```python
from build123d import *

# Parameters (mm, degrees)
SKETCH1_R           = 57
BOSS_EXTRUDE1_DEPTH = 38
SKETCH2_R           = 51
CUT_EXTRUDE1_DEPTH  = 39
SKETCH4_R           = 1.5
CUT_EXTRUDE3_DEPTH  = 15


with BuildPart() as part:
    # Sketch1 → Boss-Extrude1 (new body)
    with BuildSketch(Plane.XY):
        Circle(SKETCH1_R)
    extrude(amount=BOSS_EXTRUDE1_DEPTH)

    # Sketch2 → Cut-Extrude1 (cut)
    with BuildSketch(Plane.XY.offset(38)):
        Circle(SKETCH2_R)
    extrude(amount=-CUT_EXTRUDE1_DEPTH, mode=Mode.SUBTRACT)

    # Sketch4 → Cut-Extrude3 (cut)
    with BuildSketch(Plane(origin=(0, 0, 0), x_dir=(-1, 0, 0), z_dir=(0, 0, -1))):
        with Locations((0, 54)):
            Circle(SKETCH4_R)
        with Locations((54, 0)):
            Circle(SKETCH4_R)
        with Locations((0, -54)):
            Circle(SKETCH4_R)
        with Locations((-54, 0)):
            Circle(SKETCH4_R)
    cut_extrude3 = extrude(amount=-CUT_EXTRUDE3_DEPTH, mode=Mode.SUBTRACT)

    # Mirror1: Cut-Extrude3 across plane
    add(cut_extrude3.mirror(Plane.XY.offset(19)), mode=Mode.SUBTRACT)


solid = part.part
```
Geometry: final body of the model. Coordinates: model frame, mm. A direction names the side the tool comes from. Give positions to 0.01 mm unless a question says otherwise; leave off trailing zeros. Loops run counter-clockwise (first coordinate to the right, second up) from the corner with the lowest first, then second, coordinate; pieces in that order, holes last. Notation, with made-up numbers: (-7, 76.25) -> (24, 76.25) arc R8 ccw to (24, 88.25) -> close; hole circle Ø2 at (14.5, -4). An arc over 180 degrees is marked (long way). Use one line per item in the form item = value.
Item 1: Line query: probe 1 along Y at (x, z) = (0, 33); probe 2 along X at (y, z) = (-32.5, 31); probe 3 along Y at (x, z) = (-26.5, 13). Output: solid intervals per line, ascending.
A:
probe_1 = -57 to -55.5, -52.5 to -51, 51 to 52.5, 55.5 to 57
probe_2 = -46.83 to -39.3, 39.3 to 46.83
probe_3 = -50.47 to -43.57, 43.57 to 50.47
Item 2: Pin query (flat end, axial travel): P1, Ø2.5, axis at x = 0, y = -54, coming from the +Z side; P2, Ø1.5, axis at x = -0.5, y = -54, coming from the -Z side; P3, Ø1, axis at x = -4.5, z = 4.5, coming from the -Y side. Return the tip coordinate at first contact, or that it passes through.
A:
P1 = 23
P2 = 15
P3 = -56.86
Item 3: Draft query along X for faces 4 (the face through (55.2, -0.9, 7.4)), 5 (the face through (-21, 47, 0)), 6 (the face through (52.654, -21.831, 18.734)). Return one class per face: pulls with the +X half, pulls with the -X half, needs draft (parallel to the pull), parting line crosses it, or undercut.
A:
face_4 = undercut
face_5 = needs draft
face_6 = parting line crosses it
Item 4: Section query D-D on x = 34. Output: boundary loops of the cut face in (y, z).
A:
outline = (-45.75, 0) -> (-38.01, 0) -> (-38.01, 38) -> (-45.75, 38) -> close; (38.01, 0) -> (45.75, 0) -> (45.75, 38) -> (38.01, 38) -> close
Item 5: Section query C-C on z = 7. Output: boundary loops of the cut face in (x, y).
A:
outline = circle Ø114 at (0, 0); hole circle Ø3 at (-54, 0); hole circle Ø102 at (0, 0); hole circle Ø3 at (0, -54); hole circle Ø3 at (0, 54); hole circle Ø3 at (54, 0)
Item 6: Section query B-B on x = -43.5. Output: boundary loops of the cut face in (y, z), and give its area (3 significant figures).
A:
outline = (-36.83, 0) -> (-26.62, 0) -> (-26.62, 38) -> (-36.83, 38) -> close; (26.62, 0) -> (36.83, 0) -> (36.83, 38) -> (26.62, 38) -> close
area = 776 mm^2
Item 7: Section query A-A on y = 0. Output: boundary loops of the cut face in (x, z), and give its area (3 significant figures).
A:
outline = (-57, 0) -> (-55.5, 0) -> (-55.5, 15) -> (-52.5, 15) -> (-52.5, 0) -> (-51, 0) -> (-51, 38) -> (-52.5, 38) -> (-52.5, 23) -> (-55.5, 23) -> (-55.5, 38) -> (-57, 38) -> close; (51, 0) -> (52.5, 0) -> (52.5, 15) -> (55.5, 15) -> (55.5, 0) -> (57, 0) -> (57, 38) -> (55.5, 38) -> (55.5, 23) -> (52.5, 23) -> (52.5, 38) -> (51, 38) -> close
area = 276 mm^2
Item 8: Access query for faces 1 (the face through (-55.43, 0.45, 30.6)), 2 (the face through (54, 0, 15)), 3 (the face through (-11.056, -49.787, 19.266)). Directions: +Z, -Z, +X, -X, +Y, -Y. A direction counts if a zero-diameter tool reaches every point of the face in a straight line with its end or side. Return the directions, or none.
A:
face_1 = +Z
face_2 = -Z
face_3 = +Z, -Z
